Autodesk Inventor part; units mm, degrees
ref_plane "YZ Plane" through (0, 0, 0) normal (1, 0, 0) x (0, 1, 0)
ref_plane "XZ Plane" through (0, 0, 0) normal (0, 1, 0) x (-1, 0, 0)
ref_plane "XY Plane" through (0, 0, 0) normal (0, 0, 1) x (1, 0, 0)
sketch "Sketch1" plane through (0, 0, 0) normal (0, 1, 0) x (-1, 0, 0)
  line L0 (0, -44.45) -> (-22.25, -44.45)
  line L1 (-22.25, -44.45) -> (-22.25, -42.45)
  line L2 (-22.25, -42.45) -> (0, -42.45)
  line L3 (0, -42.45) -> (0, -44.45)
  line L4 (0, -42.45) -> (0, 0) construction
  line L5 (0, 0) -> (-22.25, 0)
  line L6 (-22.25, 0) -> (-22.25, -42.45) construction
  dimension "d0" = 2
  dimension "d1" = 22.25
  dimension "d15" = 88.9
revolve "Revolve1" add sketch "Sketch1" angle 360 about axis through (0, 0, 0) along (1, 0, 0)
sketch "Sketch2" plane through (0, 0, 0) normal (0, 1, 0) x (-1, 0, 0)
  line L0 (0, -44.45) -> (-22.25, -44.45)
  line L1 (-66.75, -44.45) -> (-89, -44.45)
  line L2 (-89, -44.45) -> (-89, -42.85)
  line L3 (-89, -42.85) -> (-66.75, -42.85)
  line L4 (-66.75, -42.85) -> (-66.75, -44.45)
  line L5 (-22.25, -44.45) -> (-66.75, -44.45) construction
  line L6 (-66.75, -42.85) -> (-66.75, -6.4) construction
  line L7 (-66.75, -6.4) -> (-89, -6.4) construction
  line L8 (-89, -6.4) -> (-89, -42.85) construction
  dimension "d2" = 44.5
  dimension "d4" = 1.6
  dimension "d5" = 22.25
  dimension "d16" = 76.1
revolve "Revolve2" add sketch "Sketch2" angle 360 about axis through (66.75, 0, -6.4) along (1, 0, 0)
sketch "Sketch3" plane through (66.75, 0, -6.4) normal (-1, 0, 0) x (0, 0, 1)
  circle A0 centre (0, 0) radius 38.05
loft "Loft1" add profiles "Sketch3" section 1 edges at (22.25, 0, 44.45)
sketch "Sketch4" plane through (22.25, 0, 0) normal (-1, 0, 0) x (0, 0, 1)
  circle A0 centre (0, 0) radius 42.45
  circle A1 centre (0, 0) radius 42.45
sketch "Sketch5" plane through (66.75, 0, -6.4) normal (1, 0, 0) x (0, 0, -1)
  circle A0 centre (0, 0) radius 36.45
  circle A1 centre (0, 0) radius 36.45
loft "Loft2" cut profiles "Sketch4", "Sketch5"
equation "\"d0\" = T"
equation "\"d1\" = 0.25 * L"
equation "\"d15\" = D"
equation "\"d2\" = 0.5 * L"
equation "\"d4\" = T1"
equation "\"d5\" = 0.25 * L"
equation "\"d16\" = D1"
equation "\"D\" = 88.9"
equation "\"T\" = 2"
equation "\"L\" = 89"
equation "\"D1\" = 76.1"
equation "\"T1\" = 1.6"
equation "\"Size_Designation\" = 1.2345"
properties part number "ISO 5251 Eccentric reducers DN80 x DN65 2" material "Stainless Steel"
Build history of the part. All positions in model axes, mm. A direction names the side the tool comes from. Round coordinates to 2 decimals unless told otherwise and drop trailing zeros. Loops run counter-clockwise (first coordinate to the right, second up) from the corner with the lowest first, then second, coordinate; pieces in that order, holes last.
Item 1: Saw through at A-A (x = 72). List the corners of the cut face in (y, z), then the cut area to 3 significant figures.
Item 2: Two-plate mould, pull along Z, no slides. Class faces 3 (the face through (0, -36, -23)), 4 (the face through (11.281, 13.352, -42.397)), 5 (the face through (10.97, -42.09, 5.53)): released by +Z, released by -Z, zero draft, split by the parting line, or undercut.
Item 3: Pin check, flat tips, straight feed: P1, Ø8, axis at x = 47.5, y = -5, coming from the +Z side; P2, Ø2, axis at x = 39, y = -26, coming from the -Z side; P3, Ø12, axis at x = 63, z = 24.5, coming from the -Y side. Stop position of each tip, or through.
Item 4: Which spindle directions (+Z, -Z, +X, -X, +Y, -Y) get a long thin tool onto all of the face, cutting with end or side? Do faces 1 (the face through (89, -31, -26)), 2 (the face through (78.031, 11.429, -42.693)). Say none if no direction does.
Item 5: Drill centre lines: line 1 along Y through (x, z) = (75.25, -6.4); line 2 along Z through (x, y) = (81, 0); line 3 along Y through (x, z) = (16, 0). Where is each one in solid material? Low to high.
Worked answers:
1. outline: circle Ø76.1 at (0, -6.4); hole circle Ø72.9 at (0, -6.4)
1. area: 374 mm2
2. face 3: zero draft
2. face 4: split by the parting line
2. face 5: undercut
3. P1: stops at z = 38.11
3. P2: stops at z = -36.21
3. P3: stops at y = -30.25
4. face 1: +Z, -Z, +X, +Y, -Y
4. face 2: +X
5. line 1: y = -38.05 to -36.45, 36.45 to 38.05
5. line 2: z = -44.45 to -42.85, 30.05 to 31.65
5. line 3: y = -44.45 to -42.45, 42.45 to 44.45
